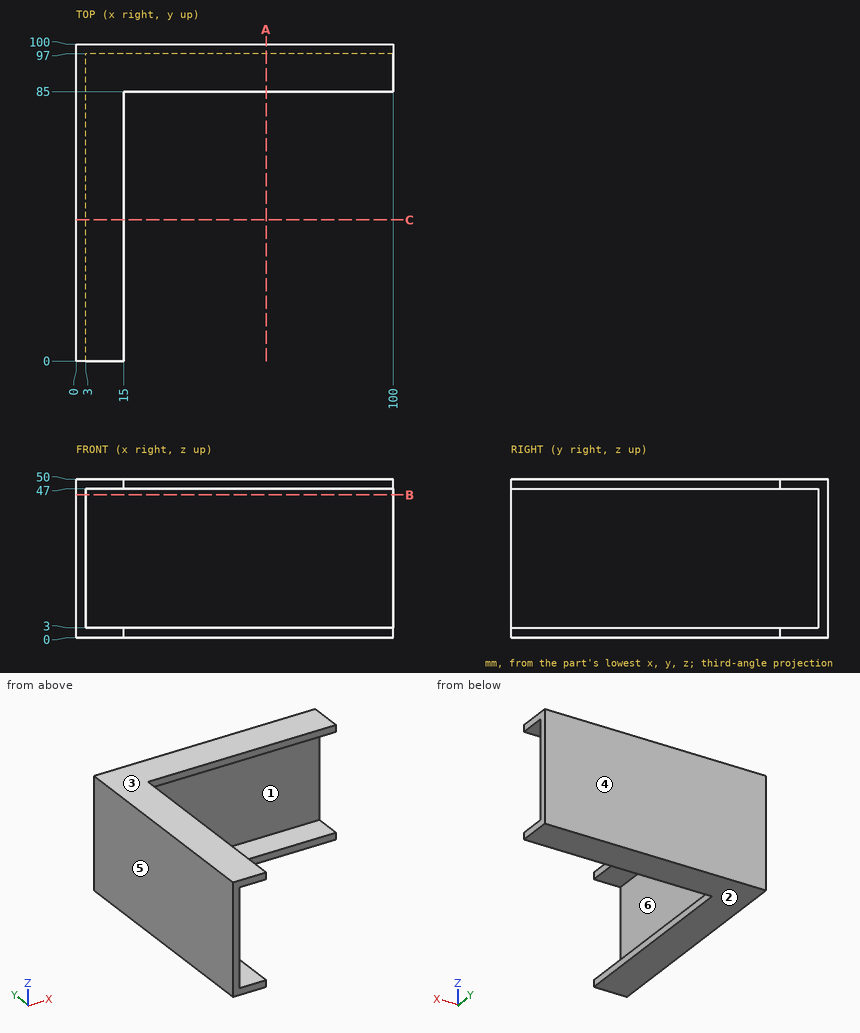
Geometry: see drawing. Coordinates: mm, zero at the bounding-box minimum. A direction names the side the tool comes from. Round coordinates to 2 decimals unless told otherwise and drop trailing zeros. Write each loop counter-clockwise with the first axis right and the second up, starting at its lowest first coordinate (ties: lowest second). Pieces come first, ordered by that corner, then holes. Notation, with made-up numbers: M -4.75,-9.75 L 30.25,-9.75 A15 ccw 30.25,16.25 Z; hole C 42,-23.5 d5. An arc over 180 degrees is marked long. Answer as a JSON object with one key per item and string values. Group by question number.
(1) Mould query, pull axis Z, two halves, no side actions, for the marked faces 1, 2, 3 and 4. Classes: +Z half, -Z half, draft (parallel to the pull), parting line (faces both ways), or undercut.
(2) Reachability of the marked faces 5 and 6 from +Z, -Z, +X, -X, +Y, -Y: full face, straight path, thin tool, end or side. Return the list, or none.
(3) Section query B-B on z = 45. Output: boundary loops of the cut face in (x, y).
(4) First-contact query: pin 1 (0.9 mm diameter, centred on y = 51.5, z = 1, fed in from +X); pin 2 (2 mm diameter, centred on x = 31, z = 42, fed in from -Y); pin 3 (3.5 mm diameter, centred on x = 72, z = 1.5, fed in from -Y). Flat tips, straight axial feed; report the tip coordinate or a pass-through.
(5) Section query A-A on x = 60. Output: boundary loops of the cut face in (y, z).
(6) Ray query, line 1 (Z direction, x = 51, y = 95.5); line 2 (Y direction, x = 86.5, z = 15); line 3 (X direction, y = 26.5, z = 15). Return the intervals inside material, ascending. Write a range as [from, to].
(7) Section query C-C on y = 44.5. Output: boundary loops of the cut face in (x, z), then the cut area to 3 significant figures.
Computed values:
{
 "1": {"face 1": "undercut", "face 2": "-Z half", "face 3": "+Z half", "face 4": "draft"},
 "2": {"face 5": "+Z, -Z, -X, +Y, -Y", "face 6": "+X, -Y"},
 "3": {"outline": "M 0,0 L 3,0 L 3,97 L 100,97 L 100,100 L 0,100 Z"},
 "4": {"pin 1": "x = 15", "pin 2": "y = 97", "pin 3": "y = 85"},
 "5": {"outline": "M 85,0 L 100,0 L 100,50 L 85,50 L 85,47 L 97,47 L 97,3 L 85,3 Z"},
 "6": {"line 1": "[0, 3], [47, 50]", "line 2": "[97, 100]", "line 3": "[0, 3]"},
 "7": {"outline": "M 0,0 L 15,0 L 15,3 L 3,3 L 3,47 L 15,47 L 15,50 L 0,50 Z", "area": "222 mm^2"}
}
